Autodesk Inventor part; units mm, degrees
ref_plane "YZ Plane" through (0, 0, 0) normal (1, 0, 0) x (0, 1, 0)
ref_plane "XZ Plane" through (0, 0, 0) normal (0, 1, 0) x (-1, 0, 0)
ref_plane "XY Plane" through (0, 0, 0) normal (0, 0, 1) x (1, 0, 0)
sketch "Sketch1" plane through (0, 0, 0) normal (0, 0, 1) x (1, 0, 0)
  line L0 (0, 0) -> (50.8, 0)
  line L1 (50.8, 0) -> (50.8, 19.05)
  line L2 (50.8, 19.05) -> (0, 19.05)
  line L3 (0, 19.05) -> (0, 0)
  dimension "d0" = 50.8
  dimension "d1" = 19.05
extrude "Extrusion1" add sketch "Sketch1" along normal blind 6.35
sketch "Sketch2" plane through (0, 0, 6.35) normal (0, 0, 1) x (1, 0, 0)
  line L0 (0, 19.05) -> (0, 0)
  line L1 (50.8, 19.05) -> (0, 19.05)
  line L2 (0, 0) -> (6.35, 0)
  line L3 (6.35, 0) -> (6.35, 19.05)
  line L4 (6.35, 19.05) -> (0, 19.05)
  line L5 (0, 19.05) -> (0, 0)
  dimension "d4" = 6.35
extrude "Extrusion2" add sketch "Sketch2" along normal blind 34.29
sketch "Sketch3" plane through (6.35, 0, 6.35) normal (1, 0, 0) x (0, 0, -1)
  line L0 (-26.67, 9.525) -> (-7.62, 9.525) construction
  line L1 (-26.67, 6.35) -> (-7.62, 6.35)
  line L2 (-7.62, 12.7) -> (-26.67, 12.7)
  arc A0 (-26.67, 12.7) -> (-26.67, 6.35) centre (-26.67, 9.525) ccw
  arc A1 (-7.62, 6.35) -> (-7.62, 12.7) centre (-7.62, 9.525) ccw
  point P0 (6.35, 0)
  point P1 (-17.145, 9.525)
  dimension "d7" = 9.525
  dimension "d8" = 6.35
extrude "Extrusion3" cut sketch "Sketch3" against normal blind 34.29
sketch "Sketch4" plane through (0, 0, 6.35) normal (0, 0, 1) x (1, 0, 0)
  line L0 (44.45, 9.525) -> (12.7, 9.525) construction
  line L1 (44.45, 12.7) -> (12.7, 12.7)
  line L2 (12.7, 6.35) -> (44.45, 6.35)
  arc A0 (44.45, 6.35) -> (44.45, 12.7) centre (44.45, 9.525) ccw
  arc A1 (12.7, 12.7) -> (12.7, 6.35) centre (12.7, 9.525) ccw
  point P0 (0, 0)
  point P1 (28.575, 9.525)
  dimension "d11" = 15.875
  dimension "d12" = 6.35
extrude "Extrusion4" cut sketch "Sketch4" against normal blind 34.29
fillet "Fillet1" radius 3.175 1 edges at (6.35, 9.525, 6.35)
sketch "Sketch5" plane through (50.8, 0, 0) normal (1, 0, 0) x (0, 0, -1)
  line L0 (0, 19.05) -> (-40.64, 19.05)
  line L1 (0, 19.05) -> (-41.8279, 19.05)
  line L2 (-41.8279, 19.05) -> (-41.8279, 18.0326)
  line L3 (-41.8279, 18.0326) -> (0, 18.0326)
  line L4 (0, 18.0326) -> (0, 19.05)
  line L5 (0, 19.05) -> (0, 0)
  line L6 (-40.64, 0) -> (-40.64, 19.05)
  line L7 (0, 0) -> (-40.64, 0)
  line L8 (-40.64, 0) -> (-40.64, 1.0192)
  line L9 (-40.64, 1.0192) -> (0, 1.0192)
  line L10 (0, 1.0192) -> (0, 0)
extrude "Extrusion5" cut sketch "Sketch5" against normal through all contours L4 L3 L6 L0 | L6 L3 L2 L1 | L5 L7 L6 L9
sketch "Sketch6" plane through (0, 0, 0) normal (0, 0, -1) x (-1, 0, 0)
  line L0 (-50.8, 18.0326) -> (-9.525, 18.0326)
  line L1 (-25.4, 18.0326) -> (-61.3669, 18.0326)
  line L2 (-61.3669, 18.0326) -> (-61.3669, -3.7914)
  line L3 (-61.3669, -3.7914) -> (-25.4, -3.7914)
  line L4 (-25.4, -3.7914) -> (-25.4, 18.0326)
  point P0 (0, 0)
extrude "Extrusion6" cut sketch "Sketch6" against normal through all
properties part number "BLKbackplaneBracketMid"
Design review of the part built by this model. Coordinates are the model's own, in mm. A direction names the side the tool comes from. Give positions to 0.01 mm unless a question says otherwise; leave off trailing zeros. Write each loop counter-clockwise with the first axis right and the second up, starting at its lowest first coordinate (ties: lowest second). Pieces come first, ordered by that corner, then holes. Notation, with made-up numbers: M -14.75,19.25 L -0.75,19.25 A14 ccw -0.75,31.25 Z; hole C 39,-12.75 d11. An arc over 180 degrees is marked long. Answer as a JSON object with one key per item and string values. Group by question number.
1) For line 1 along Y through (x, z) = (1.5, 31); line 2 along X through (y, z) = (17, 20.5), list the stretches that pass through material, from the lowest coordinate up.
2) Mouldability with a two-part tool opening along Y and no side actions: class faces 5 (the face through (3.219, 9.455, 10.796)), 6 (the face through (7.3, 9.64, 7.26)), 7 (the face through (19, 6.35, 3)), 8 (the face through (5, 1.019, 16)) as released by +Y, released by -Y, zero draft, split by the parting line, or undercut.
3) We need section A-A (x = 1.5). Give the boundary of the cut face in (y, z) (3 decimals), and give its area (3 significant figures).
4) We need section D-D (x = 23.5). Give the boundary of the cut face in (y, z), and give its area (3 significant figures).
5) Tool access review of faces 1 (the face through (17, 4, 6.35)), 2 (the face through (19, 12.7, 3)), 3 (the face through (9.7, 7.8, 0)), 4 (the face through (3.219, 9.595, 36.194)): name each direction out of +Z, -Z, +X, -X, +Y, -Y from which nothing blocks a thin tool from reaching the whole face with its end or side.
6) We need section B-B (z = 3.5). Give the boundary of the cut face in (x, y) (3 decimals), and give its area (3 significant figures).
7) Clearance check with flat-ended pins moving along their axes: pin 1 Ø5 at (y, z) = (11.5, 20.5) entering from +X; pin 2 Ø3 at (y, z) = (15.5, 9) entering from +X; pin 3 Ø7 at (x, y) = (20, 13) entering from +Z; pin 4 Ø5 at (y, z) = (11, 33.5) entering from -X. State where each tip first meets the part, or that it passes through.
8) We need section C-C (z = 22). Give the boundary of the cut face in (x, y).
Answer key:
{
 "1": {"line 1": "y = 1.02 to 6.35, 12.7 to 18.03", "line 2": "x = 0 to 6.35"},
 "2": {"face 5": "undercut", "face 6": "zero draft", "face 7": "undercut", "face 8": "released by -Y"},
 "3": {"outline": "M 1.019,0 L 18.033,0 L 18.033,40.64 L 1.019,40.64 Z; hole M 6.35,13.97 A3.175 ccw 12.7,13.97 L 12.7,33.02 A3.175 ccw 6.35,33.02 Z", "area": "539 mm²"},
 "4": {"outline": "M 1.02,0 L 6.35,0 L 6.35,6.35 L 1.02,6.35 Z; M 12.7,0 L 18.03,0 L 18.03,6.35 L 12.7,6.35 Z", "area": "67.7 mm²"},
 "5": {"face 1": "+Z, +X, +Y, -Y", "face 2": "+Z, -Z, +X", "face 3": "-Z, +X, -X, +Y, -Y", "face 4": "+X, -X"},
 "6": {"outline": "M 0,1.019 L 25.4,1.019 L 25.4,6.35 L 12.7,6.35 A3.175 cw 12.7,12.7 L 25.4,12.7 L 25.4,18.033 L 0,18.033 Z", "area": "336 mm²"},
 "7": {"pin 1": "stops at x = 6.35", "pin 2": "stops at x = 7.08", "pin 3": "stops at z = 6.35", "pin 4": "stops at x = 0"},
 "8": {"outline": "M 0,1.02 L 6.35,1.02 L 6.35,6.35 L 0,6.35 Z; M 0,12.7 L 6.35,12.7 L 6.35,18.03 L 0,18.03 Z"}
}
